Input: part model. Units: mm. Frame: model coordinates. A direction names the side the tool comes from. Round coordinates to 2 decimals unless told otherwise and drop trailing zeros. Write each loop counter-clockwise with the first axis right and the second up, starting at its lowest first coordinate (ties: lowest second). Pieces come first, ordered by that corner, then holes. Notation, with made-up numbers: (-19, 73) -> (22, 73) arc R27 cw to (22, 109) -> close; hole circle Ø4 at (2.5, 36). An arc over 180 degrees is marked (long way). Use CSV: the item, a comma, the result in double quotes.
Autodesk Inventor part; units mm, degrees
ref_plane "YZ Plane" through (0, 0, 0) normal (1, 0, 0) x (0, 1, 0)
ref_plane "XZ Plane" through (0, 0, 0) normal (0, 1, 0) x (-1, 0, 0)
ref_plane "XY Plane" through (0, 0, 0) normal (0, 0, 1) x (1, 0, 0)
sketch "Skizze1" plane through (0, 0, 0) normal (0, 0, 1) x (1, 0, 0)
  line L0 (-30, 0) -> (30, 0)
  line L1 (30, 0) -> (30, 2)
  line L2 (30, 2) -> (24.75, 2)
  line L3 (24.75, 2) -> (24.75, 3.5)
  line L4 (24.75, 3.5) -> (25.75, 3.5)
  line L5 (25.75, 3.5) -> (24, 7)
  line L6 (24, 7) -> (22, 7)
  line L7 (22, 7) -> (22, 2)
  line L8 (22, 2) -> (-22, 2)
  line L9 (-22, 2) -> (-22, 7)
  line L10 (-22, 7) -> (-24, 7)
  line L11 (-24, 7) -> (-25.75, 3.5)
  line L12 (-25.75, 3.5) -> (-24.75, 3.5)
  line L13 (-24.75, 3.5) -> (-24.75, 2)
  line L14 (-24.75, 2) -> (-30, 2)
  line L15 (-30, 2) -> (-30, 0)
  point P0 (0, 0)
  point P1 (0, 0)
  dimension "d0" = 49.5
  dimension "d1" = 24.75
  dimension "d2" = 5.25
  dimension "d3" = 5.25
  dimension "d4" = 1
  dimension "d5" = 1
  dimension "d6" = 44
  dimension "d7" = 2
  dimension "d8" = 22
  dimension "d9" = 2
  dimension "d10" = 5
  dimension "d11" = 2
  dimension "d12" = 2
  dimension "d13" = 1.5
extrude "Extrusion1" add sketch "Skizze1" along normal blind 11
sketch "Skizze2" plane through (30, 0, 0) normal (1, 0, 0) x (0, 0, -1)
  line L0 (-11, 0) -> (-11, 2)
  line L1 (-19, 0) -> (-19, -9)
  line L2 (-19, -9) -> (-15, -9)
  line L3 (-15, -9) -> (-15, -7)
  line L4 (-15, -7) -> (-17, -7)
  line L5 (-17, -7) -> (-17, -5)
  line L6 (-17, -5) -> (-15, -5)
  line L7 (-15, -5) -> (-15, 0)
  line L8 (0, 0) -> (-11, 0)
  line L9 (-11, 2) -> (-11, 0)
  line L10 (-15, 0) -> (-11, 0)
  line L11 (-11, 2) -> (-11, 7)
  line L12 (-11, 0) -> (-11, 2)
  line L13 (-11, 2) -> (-19, 2)
  line L14 (-19, 2) -> (-19, 0)
  point P0 (-11, 1)
  dimension "d16" = 9
  dimension "d17" = 4
  dimension "d18" = 2
  dimension "d19" = 2
  dimension "d20" = 2
  dimension "d23" = 4
  dimension "d24" = 2
extrude "Extrusion2" add sketch "Skizze2" against normal up to surface (60 mm away)
sketch "Skizze3" plane through (30, -5, 15) normal (0, 0, -1) x (-1, 0, 0)
  line L0 (60, 7) -> (60, -4)
  line L1 (0, 0) -> (60, 0)
  line L2 (60, -4) -> (58.5, -4)
  line L3 (58.5, -4) -> (58.5, 0)
  line L4 (58.5, 0) -> (60, 0)
  line L5 (60, 0) -> (60, -4)
  line L6 (0, 7) -> (0, -4)
  line L7 (0, -4) -> (1.5, -4)
  line L8 (1.5, -4) -> (1.5, 0)
  line L9 (1.5, 0) -> (0, 0)
  line L10 (0, 0) -> (0, -4)
  line L11 (60, 5) -> (0, 5)
  point P0 (30, 5)
  point P1 (30, 5)
  point P2 (1.5, 0)
  dimension "d25" = 57
  dimension "d26" = 28.5
extrude "Extrusion3" add sketch "Skizze3" against normal up to surface (2 mm away) contours L0 L2 L3 L1 | L1 L8 L7 L6
sketch "Skizze4" plane through (-30, 0, 0) normal (0, -1, 0) x (1, 0, 0)
  line L0 (52, 0) -> (8, 0)
  line L1 (20, 0) -> (40, 0)
  line L2 (40, 0) -> (40, 4)
  line L3 (40, 4) -> (20, 4)
  line L4 (20, 4) -> (20, 0)
  line L5 (20, 4) -> (18, 4)
  line L6 (18, 4) -> (18, 1.8)
  line L7 (18, 1.8) -> (20, 1.8)
  line L8 (20, 1.8) -> (20, 4)
  line L9 (40, 4) -> (42, 4)
  line L10 (42, 4) -> (42, 1.8)
  line L11 (42, 1.8) -> (40, 1.8)
  line L12 (40, 1.8) -> (40, 4)
  point P0 (30, 0)
  point P1 (40, 2.9)
  point P2 (41, 1.8)
  point P3 (30, 0)
  dimension "d29" = 20
  dimension "d30" = 2
  dimension "d31" = 2
  dimension "d32" = 2.2
  dimension "d33" = 1.8
  dimension "d34" = 10
extrude "Extrusion4" cut sketch "Skizze4" against normal blind 10
sketch "Skizze5" plane through (30, -9, 15) normal (0, 0, -1) x (-1, 0, 0)
  line L0 (0, 11) -> (0, 0)
  line L1 (0, 9) -> (60, 9)
  line L2 (0, 5) -> (4, 5)
  line L3 (4, 5) -> (4, 9)
  line L4 (4, 9) -> (0, 9)
  line L5 (0, 9) -> (0, 5)
  line L6 (60, 0) -> (60, 9)
  line L7 (60, 5) -> (56, 5)
  line L8 (56, 5) -> (56, 9)
  line L9 (56, 9) -> (60, 9)
  line L10 (60, 9) -> (60, 5)
  point P0 (30, 9)
  dimension "d37" = 4
  dimension "d38" = 4
  dimension "d39" = 4
extrude "Extrusion5" cut sketch "Skizze5" against normal blind 10
equation "\"d3\" = d2"
equation "\"d5\" = d4"
equation "\"d9\" = d7"
equation "\"d31\" = d30"
equation "\"d38\" = d37"
equation "\"d39\" = d37"
properties part number "Clip"
Item 1: Section query C-C on z = 17.75. Return the cut outline in (x, y), plus the area to 3 significant figures.
Worked answers:
outline,"(-30, -9) -> (30, -9) -> (30, -4) -> (26, -4) -> (26, 0) -> (30, 0) -> (30, 2) -> (-30, 2) -> (-30, 0) -> (-26, 0) -> (-26, -4) -> (-30, -4) -> close"
area,"628 mm²"
Item 2: Pull-direction query (X, two-part tool) for faces 5 (the face through (-10, 1, 1)), 6 (the face through (0, 1, 4)), 7 (the face through (0, -9, 17)), 8 (the face through (-30, 1, 9)); classes: +X half, -X half, draft (parallel to the pull), parting line (faces both ways), or undercut.
Worked answers:
face 5,"undercut"
face 6,"undercut"
face 7,"draft"
face 8,"-X half"
Item 3: Line query: line 1 (X direction, y = 2.25, z = 1.25); line 2 (Y direction, x = -9, z = 5); line 3 (Z direction, x = -2, y = -7.75). Output: solid intervals per line, ascending.
Worked answers:
line 1,"x = -24.75 to -22, 22 to 24.75"
line 2,"y = 0 to 2"
line 3,"z = 15 to 19"
Item 4: Section query D-D on y = -1. Return the cut outline in (x, z), plus the area to 3 significant figures.
Worked answers:
outline,"(-26, 15) -> (26, 15) -> (26, 19) -> (-26, 19) -> close"
area,"208 mm²"
Item 5: First-contact query: pin 1 Ø10 at (x, z) = (3, 7) entering from +Y; pin 2 Ø6 at (y, z) = (5.5, 9.5) entering from -X; pin 3 Ø1.6 at (x, y) = (-12, -6.5) entering from -Z. Flat tips, straight axial feed; report the tip coordinate or a pass-through.
Worked answers:
pin 1,"stops at y = 2"
pin 2,"stops at x = -25.75"
pin 3,"stops at z = 15"
Item 6: Section query A-A on z = 3. Return the cut outline in (x, y), plus the area to 3 significant figures.
Worked answers:
outline,"(-30, 0) -> (-12, 0) -> (-12, 2) -> (-22, 2) -> (-22, 7) -> (-24, 7) -> (-25.75, 3.5) -> (-24.75, 3.5) -> (-24.75, 2) -> (-30, 2) -> close; (12, 0) -> (30, 0) -> (30, 2) -> (24.75, 2) -> (24.75, 3.5) -> (25.75, 3.5) -> (24, 7) -> (22, 7) -> (22, 2) -> (12, 2) -> close"
area,"100 mm²"
Item 7: Section query B-B on x = -15. Return the cut outline in (y, z), plus the area to 3 significant figures.
Worked answers:
outline,"(-9, 15) -> (-7, 15) -> (-7, 17) -> (-5, 17) -> (-5, 15) -> (0, 15) -> (0, 0) -> (2, 0) -> (2, 19) -> (-9, 19) -> close"
area,"70.0 mm²"
Item 8: Set-up query: faces 1 (the face through (-26, -2, 17)), 2 (the face through (0.4, -4.6, 15)), 3 (the face through (23, 5, 11)), 4 (the face through (-12, 1, 3)). Return all of +Z, -Z, +X, -X, +Y, -Y with unobstructed straight access to the full face (end or side cutting, diameter ignored); none if empty.
Worked answers:
face 1,"+Z, -Z, -X"
face 2,"-Z, +X, -X, -Y"
face 3,"+Z, +X, -X, +Y"
face 4,"+Y, -Y"
